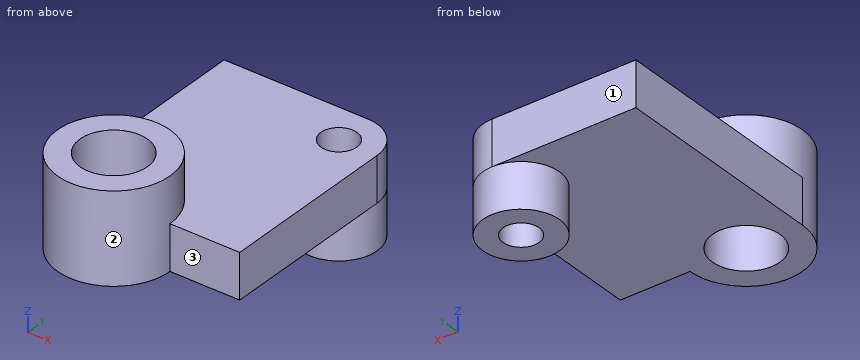
from build123d import *
from build123d.topology import SkipClean

# Parameters (mm, degrees)
SKETCH_1_R          = 4
EXTRUDE_1_DEPTH     = 10
CUT_EXTRUDE_1_DEPTH = 63.713634881
SKETCH_3_R          = 12.5
EXTRUDE_2_DEPTH     = 10
CUT_EXTRUDE_2_REACH = 64.292
SKETCH_4_R          = 7.5
EXTRUDE_START       = 10
SKETCH_5_R          = 12.5
SKETCH_5_R_2        = 7.5
EXTRUDE_3_DEPTH     = 10
SKETCH_6_R          = 8.5
SKETCH_6_R_2        = 4
EXTRUDE_4_DEPTH     = 10
EXTRUDE_START_2     = -10
EXTRUDE_5_DEPTH     = 10
CUT_EXTRUDE_3_DEPTH = 65.654852873


with BuildPart() as part:
    # Эскиз1 → Бобышка-Вытянуть1 (new body)
    with BuildSketch(Plane.XY):
        with BuildLine():
            Line((13, -15), (8.188495856, 2.280029742))
            ThreePointArc((8.188495856, 2.280029742), (2.584908604, 8.097422276), (-5.352868863, 6.602786907))
            Line((-5.352868863, 6.602786907), (-32, -15))
            Line((-32, -15), (-32, -40))
            Line((-32, -40), (-13, -40))
            ThreePointArc((-13, -40), (0, -53), (13, -40))
            Line((13, -40), (13, -15))
        make_face()
        Circle(SKETCH_1_R, mode=Mode.SUBTRACT)
    extrude(amount=EXTRUDE_1_DEPTH)

    # Эскиз2 → Вырез-Вытянуть1 (cut, through all)
    with BuildSketch(Plane.XY.offset(10)):
        with BuildLine():
            Line((-13, -40), (13, -40))
            ThreePointArc((13, -40), (0, -53), (-13, -40))
        make_face()
    extrude(amount=-CUT_EXTRUDE_1_DEPTH, mode=Mode.SUBTRACT)

    # Эскиз3 → Бобышка-Вытянуть2 (add)
    with BuildSketch(Plane.XY.offset(10)):
        with Locations((-19.5, -40)):
            Circle(SKETCH_3_R)
    extrude(amount=-EXTRUDE_2_DEPTH)

    # Эскиз4 → Вырез-Вытянуть2 (cut, up to next)
    with BuildSketch(Plane.XY.offset(10), mode=Mode.PRIVATE) as cut_extrude_2_sk1:
        with Locations((-19.5, -40)):
            Circle(SKETCH_4_R)
    cut_extrude_2_tool1 = extrude(cut_extrude_2_sk1.sketch, amount=-CUT_EXTRUDE_2_REACH, mode=Mode.PRIVATE) & part.part
    add(cut_extrude_2_tool1.solids().sort_by_distance((-19.5, -40, 10))[0], mode=Mode.SUBTRACT)

    # Эскиз5 → Бобышка-Вытянуть3 (add)
    with BuildSketch(Plane.XY.offset(10).offset(EXTRUDE_START)):
        with Locations((-19.5, -40)):
            Circle(SKETCH_5_R)
        with Locations((-19.5, -40)):
            Circle(SKETCH_5_R_2, mode=Mode.SUBTRACT)
    extrude(amount=-EXTRUDE_3_DEPTH)

    # Эскиз6 → Бобышка-Вытянуть4 (add)
    with SkipClean():  # the faces are left unmerged after this step: merging them gives an invalid solid
        with BuildSketch(Plane(origin=(0, 0, 0), x_dir=(-1, 0, 0), z_dir=(0, 0, -1)).offset(EXTRUDE_START)):
            Circle(SKETCH_6_R)
            Circle(SKETCH_6_R_2, mode=Mode.SUBTRACT)
        extrude(amount=-EXTRUDE_4_DEPTH)

    # Эскиз7 → Бобышка-Вытянуть5 (add)
    with SkipClean():  # the faces are left unmerged after this step: merging them gives an invalid solid
        with BuildSketch(Plane.XY.offset(10).offset(EXTRUDE_START_2)):
            with BuildLine():
                Line((-32, 8.5), (-32, -15))
                Line((-32, -15), (-5.352868863, 6.602786907))
                ThreePointArc((-5.352868863, 6.602786907), (-2.839569604, 8.011669268), (4e-08, 8.5))
                Line((4e-08, 8.5), (-32, 8.5))
            make_face()
            with BuildLine():
                Line((13, 8.5), (4e-08, 8.5))
                ThreePointArc((4e-08, 8.5), (5.14148556, 6.768687187), (8.188495856, 2.280029742))
                Line((8.188495856, 2.280029742), (13, -15))
                Line((13, -15), (13, 8.5))
            make_face()
        extrude(amount=EXTRUDE_5_DEPTH)
    add(part.part.scale(1), mode=Mode.REPLACE)  # the faces are merged on a copy

    # Эскиз8 → Вырез-Вытянуть3 (cut, through all)
    with BuildSketch(Plane(origin=(0, 0, 0), x_dir=(-1, 0, 0), z_dir=(0, 0, -1))):
        with BuildLine():
            Line((-8.5, -40), (-8.5, 0))
            ThreePointArc((-8.5, 0), (-6.01040764, 6.01040764), (0, 8.5))
            Line((0, 8.5), (-13, 8.5))
            Line((-13, 8.5), (-13, -40))
            Line((-13, -40), (-8.5, -40))
        make_face()
    extrude(amount=-CUT_EXTRUDE_3_DEPTH, mode=Mode.SUBTRACT)


solid = part.part
Could you check a few things on this model? Use its own coordinates, in mm. Face numbers are marked on the shaded views. A direction names the side the tool comes from. Coordinates: 2 decimals unless noted, no trailing zeros. Loops run counter-clockwise (first coordinate to the right, second up) from the corner with the lowest first, then second, coordinate; pieces in that order, holes last. Notation, with made-up numbers: (23.5, -20.5) -> (40.5, -20.5) arc R20 cw to (40.5, -8.5) -> close; hole circle Ø6 at (68, 78). An arc over 180 degrees is marked (long way). Answer in a Markdown table with one row per item.
(1) Imagine slicing it at C-C (x = -15). List the corners of the cut face in (y, z) for me.
Results found:
| item | result |
|---|---|
| outline | (-51.66, 0) -> (-46, 0) -> (-46, 20) -> (-51.66, 20) -> close; (-34, 0) -> (8.5, 0) -> (8.5, 10) -> (-28.34, 10) -> (-28.34, 20) -> (-34, 20) -> close |
(2) Will these pins go through, and if not, where does the flat tip stop? pin 1 Ø11 at (x, z) = (0.5, 4) entering from -Y; pin 2 Ø12 at (x, z) = (-17.5, -3) entering from -Y; pin 3 Ø20 at (x, y) = (-21, -19.5) entering from -Z; pin 4 Ø5 at (x, y) = (0, 0) entering from -Z.
Results found:
| item | result |
|---|---|
| pin 1 | stops at y = -40 |
| pin 2 | stops at y = -52.5 |
| pin 3 | stops at z = 0 |
| pin 4 | passes through |
(3) Imagine slicing it at A-A (z = 2.5). List the corners of the cut face in (x, y) for me, plus the area to 3 significant figures.
Results found:
| item | result |
|---|---|
| outline | (-32, -40) arc R12.5 ccw to (-7, -40) -> (8.5, -40) -> (8.5, 0) arc R8.5 ccw to (0, 8.5) -> (-32, 8.5) -> close; hole circle Ø15 at (-19.5, -40); hole circle Ø8 at (0, 0) |
| area | 1,970 mm^2 |
(4) For the marked faces 1, 2 and 3, which set-ups out of +Z, -Z, +X, -X, +Y, -Y let a thin tool reach every point of the face, with its end or its side?
Results found:
| item | result |
|---|---|
| face 1 | +Z, -Z, +X, -X, +Y |
| face 2 | +Z |
| face 3 | +Z, -Z, +X, -Y |
(5) Imagine slicing it at B-B (x = -19.5). List the corners of the cut face in (y, z) for me.
Results found:
| item | result |
|---|---|
| outline | (-52.5, 0) -> (-47.5, 0) -> (-47.5, 20) -> (-52.5, 20) -> close; (-32.5, 0) -> (8.5, 0) -> (8.5, 10) -> (-27.5, 10) -> (-27.5, 20) -> (-32.5, 20) -> close |
(6) Imagine slicing it at D-D (y = -15.5). List the corners of the cut face in (x, z) for me, plus the area to 3 significant figures.
Results found:
| item | result |
|---|---|
| outline | (-32, 0) -> (8.5, 0) -> (8.5, 10) -> (-32, 10) -> close |
| area | 405 mm^2 |
(7) If I drill on probe 1 along Y at (x, z) = (0, -7.5); probe 2 along Y at (x, z) = (0, 6.25); probe 3 along Z at (x, y) = (-29, -4.5), over which ranges is the centre line in solid material (lowest first)?
Results found:
| item | result |
|---|---|
| probe 1 | y = -8.5 to -4, 4 to 8.5 |
| probe 2 | y = -40 to -4, 4 to 8.5 |
| probe 3 | z = 0 to 10 |
